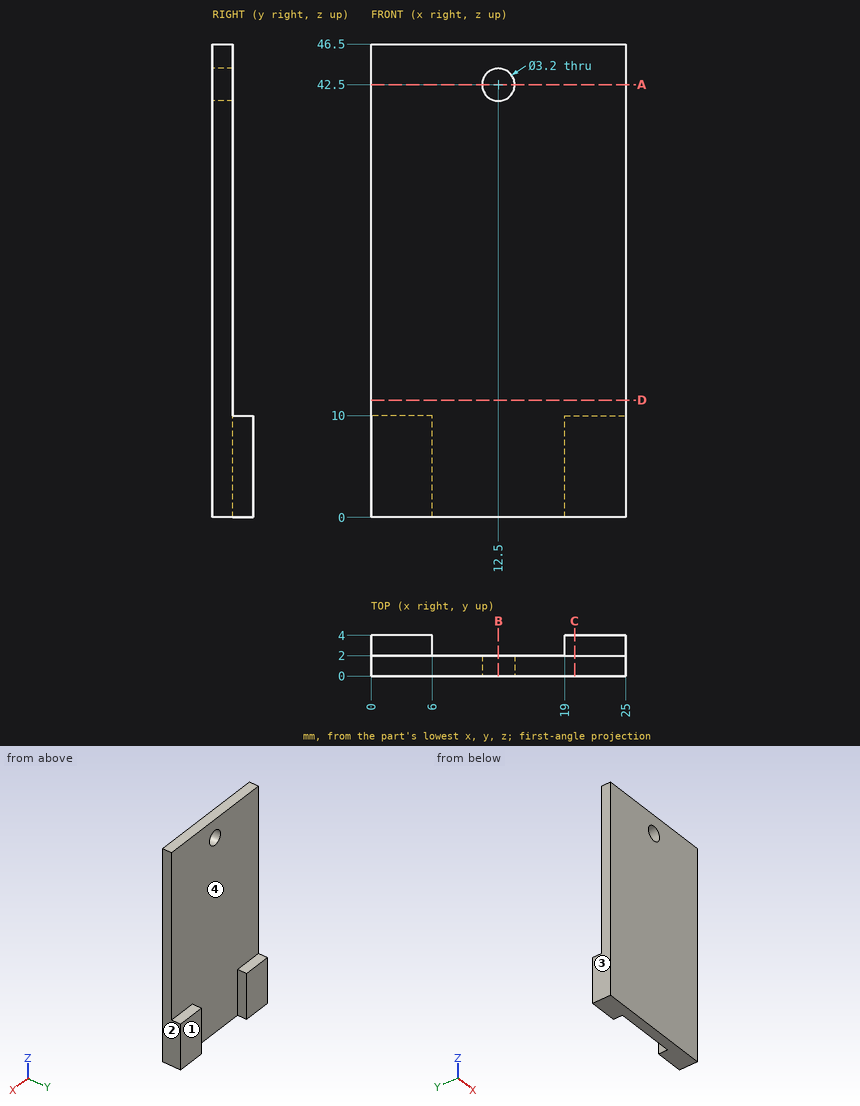
Study the drawing (mm; zero at the part's minimum x, y, z) and answer. Round coordinates to 2 decimals unless told otherwise and drop trailing zeros. Loops run counter-clockwise (first coordinate to the right, second up) from the corner with the lowest first, then second, coordinate; pieces in that order, holes last. Notation, with made-up numbers: (48, 48.5) -> (70, 48.5) arc R24 cw to (70, 77.5) -> close; hole circle Ø8 at (69.5, 35). An arc over 180 degrees is marked (long way). One line per item, written item: value.
1) A cutting plane is placed at D-D (z = 11.5). Determine the outline of the cut face in (x, y), and give its area (3 significant figures).
Answer list:
outline: (0, 0) -> (25, 0) -> (25, 2) -> (0, 2) -> close
area: 50.0 mm²
2) A cutting plane is placed at A-A (z = 42.5). Determine the outline of the cut face in (x, y), and give its area (3 significant figures).
Answer list:
outline: (0, 0) -> (10.9, 0) -> (10.9, 2) -> (0, 2) -> close; (14.1, 0) -> (25, 0) -> (25, 2) -> (14.1, 2) -> close
area: 43.6 mm²
3) The mould has two halves that part along X. Classify the marked faces 1, 2, 3 and 4: pulls with the +X half, pulls with the -X half, needs draft (parallel to the pull), parting line crosses it, or undercut.
Answer list:
face 1: needs draft
face 2: pulls with the +X half
face 3: pulls with the -X half
face 4: undercut
4) Flat-ended cylindrical pins translate along their axes: P1, Ø2, axis at x = 23.5, y = 3.5, coming from the +Z side; P2, Ø1.5, axis at y = 3, z = 31, coming from the +X side; P3, Ø4, axis at x = 12.5, z = 42.5, coming from the -Y side; P4, Ø12.5, axis at x = 9, z = 30.5, coming from the +Y side. Find the tip coordinate at first contact, or state that the pin passes through.
Answer list:
P1: stops at z = 10
P2: passes through
P3: stops at y = 0
P4: stops at y = 2
5) Consider L1, parallel to Z at x = 12.5, y = 1.5; L2, parallel to X at y = 1.3, z = 42.5; L3, parallel to X at y = 2.6, z = 5.5. Determine where each line is inside the solid, lowest interval first. Write a range as [from, to].
Answer list:
L1: z = [0, 40.9], [44.1, 46.5]
L2: x = [0, 10.9], [14.1, 25]
L3: x = [0, 6], [19, 25]
6) A cutting plane is placed at C-C (x = 20). Determine the outline of the cut face in (y, z).
Answer list:
outline: (0, 0) -> (4, 0) -> (4, 10) -> (2, 10) -> (2, 46.5) -> (0, 46.5) -> close
7) A cutting plane is placed at B-B (x = 12.5). Determine the outline of the cut face in (y, z), and give its area (3 significant figures).
Answer list:
outline: (0, 0) -> (2, 0) -> (2, 40.9) -> (0, 40.9) -> close; (0, 44.1) -> (2, 44.1) -> (2, 46.5) -> (0, 46.5) -> close
area: 86.6 mm²
